Autodesk Inventor part; units mm, degrees
ref_plane "YZ Plane" through (0, 0, 0) normal (1, 0, 0) x (0, 1, 0)
ref_plane "XZ Plane" through (0, 0, 0) normal (0, 1, 0) x (-1, 0, 0)
ref_plane "XY Plane" through (0, 0, 0) normal (0, 0, 1) x (1, 0, 0)
sketch "スケッチ2" plane through (0, 0, 0) normal (0, 0, 1) x (1, 0, 0)
  circle A0 centre (24.8946, 24.5696) radius 0.85
  circle A1 centre (3.8946, 24.5696) radius 0.85
  circle A2 centre (3.8946, 3.5696) radius 0.85
  circle A3 centre (24.8946, 24.5696) radius 2.5
  circle A4 centre (24.8946, 24.5696) radius 1.1
  circle A5 centre (3.8946, 24.5696) radius 1.1
  circle A6 centre (3.8946, 24.5696) radius 2.5
  circle A7 centre (3.8946, 3.5696) radius 2.5
  circle A8 centre (3.8946, 3.5696) radius 1.1
  line L0 (24.8946, 27.0696) -> (3.8946, 27.0696)
  line L1 (24.8946, 22.0696) -> (3.8946, 22.0696)
  line L2 (6.3946, 24.5696) -> (6.3946, 3.5696)
  line L3 (3.8946, 27.0696) -> (-21.1054, 27.0696)
  arc A9 (-21.1054, 27.0696) -> (-56.0009, 1.0696) centre (-21.1054, -9.3477) ccw
  line L4 (3.8946, 1.0696) -> (-56.0009, 1.0696) construction
  circle A10 centre (-53.6054, 0.3545) radius 2.5
  arc A11 (1.5492, 2.7041) -> (-51.1781, -0.2441) centre (-24.3623, -6.8571) ccw
  circle A12 centre (-25.9042, 23.7232) radius 3 construction
  circle A13 centre (-53.6054, 0.3545) radius 1.1
  circle A14 centre (-25.9042, 23.7232) radius 1.1
  circle A15 centre (-43.3948, 16.3537) radius 2.3971 construction
  line L5 (-43.3948, 16.3537) -> (-25.9042, 23.7232) construction
  line L6 (-43.3948, 16.3537) -> (-53.6054, 0.3545) construction
  circle A16 centre (-43.3948, 16.3537) radius 1.1
  point P0 (0, 0)
  point P1 (3.8946, 1.0696)
  point P2 (1.4587, 3.0071)
  point P3 (-51.2099, 1.0696)
  point P4 (-55.9852, 1.6541)
  point P5 (6.3946, 22.0696)
  point P6 (-25.9042, 20.719)
  dimension "d10" = 5
  dimension "d11" = 2.2
  dimension "d12" = 2.2
  dimension "d13" = 5
  dimension "d14" = 5
  dimension "d15" = 2.2
  dimension "d16" = 25
  dimension "d17" = 5
  dimension "d21" = 60
  dimension "d23" = 6
  dimension "d24" = 2.2
  dimension "d25" = 2.2
  dimension "d26" = 2.2
extrude "押し出し1" add sketch "スケッチ2" along normal blind 1.5 contours A3 | A3 L1 L2 A6 L0 | A6 | A6 L1 L2 A7 A11 A10 A9 L3 | L1 A6 L2 | A7 | A10
fillet "フィレット1" radius 2 1 edges at (6.3946, 22.0696, 0.75)
sketch "スケッチ3" plane through (0, 0, 1.5) normal (0, 0, 1) x (1, 0, 0)
  line L0 (-24.3623, 22.7621) -> (4.3946, 22.7621)
  line L1 (4.3946, 22.7621) -> (4.3946, 6.0191)
  line L2 (6.3946, 3.5696) -> (6.3946, 20.0696)
  line L3 (24.8946, 27.0696) -> (-21.1054, 27.0696)
  circle A0 centre (3.8946, 24.5696) radius 1.1
  circle A1 centre (3.8946, 24.5696) radius 2.5
  arc A2 (1.5492, 2.7041) -> (-51.1781, -0.2441) centre (-24.3623, -6.8571) ccw
  arc A3 (1.5492, 2.7041) -> (6.3946, 3.5696) centre (3.8946, 3.5696) ccw
  circle A4 centre (3.8946, 3.5696) radius 2.5
  arc A5 (3.4255, 3.3965) -> (-53.12, 0.2347) centre (-24.3623, -6.8571) ccw
  arc A6 (3.4255, 3.3965) -> (4.3946, 3.5696) centre (3.8946, 3.5696) ccw
  line L4 (4.3946, 3.5696) -> (4.3946, 20.0696)
  point P0 (0, 0)
  point P1 (2.4919, 5.639)
  point P2 (4.3946, 22.1201)
  point P3 (2.1675, 22.7621)
  dimension "d27" = 2
  dimension "d30" = 2
extrude "押し出し2" cut sketch "スケッチ3" against normal through all contours L0 A1 L1 A4 A5
fillet "フィレット2" radius 2 5 edges at (-24.3623, 22.7621, 0.75) (2.4919, 5.639, 0.75) (4.3946, 6.0191, 0.75) (4.3946, 22.1201, 0.75) (2.1675, 22.7621, 0.75)
sketch "スケッチ4" plane through (0, 0, 1.5) normal (0, 0, 1) x (1, 0, 0)
  circle A0 centre (-15.7592, 24.9158) radius 1.1
  circle A1 centre (-0.7592, 24.9158) radius 1.1
  circle A2 centre (-0.7592, 24.9158) radius 2.1538
  line L0 (24.8946, 27.0696) -> (-21.1054, 27.0696)
  line L1 (-8.969, 22.7621) -> (1.4961, 22.7621)
  line L2 (1.3946, 24.5696) -> (1.3946, 3.5696)
  point P0 (0, 0)
  dimension "d34" = 2.2
  dimension "d35" = 2.2
  dimension "d36" = 15
extrude "押し出し3" cut sketch "スケッチ4" against normal through all contours A0 | A1
properties part number "tesaki" material "アルミニウム 2014-T4"
Source: CAD feature listing. Evaluate the final solid. Frame: model axes, mm. A direction names the side the tool comes from. Round coordinates to 2 decimals unless told otherwise and drop trailing zeros. Loops run counter-clockwise (first coordinate to the right, second up) from the corner with the lowest first, then second, coordinate; pieces in that order, holes last. Notation, with made-up numbers: M -0.75,7 L 49.25,7 A20 cw 49.25,25 Z; hole C 51,58 d5. An arc over 180 degrees is marked long. Use a Markdown table: item, result. Add a question column.
1. Line query: line 1 (X direction, y = 23.75, z = 0.5); line 2 (X direction, y = 16, z = 0.6); line 3 (X direction, y = 11, z = 0.5). Output: solid intervals per line, ascending.
2. Section query A-A on y = 13.75. Return the cut outline in (x, z), then the cut area to 3 significant figures.
3. Mould query, pull axis Y, two halves, no side actions, for faces 4 (the flat face through (2, 27.07, 1)), 5 (the cylindrical face through (4.486, 23.642, 0.74)), 6 (the cylindrical face through (-3.909, 14.567, 0.76)), 7 (the cylindrical face through (6.996, 21.499, 0.76)). Classes: pulls with the +Y half, pulls with the -Y half, needs draft (parallel to the pull), parting line crosses it, or undercut.
4. Reachability of faces 1 (the flat face through (-17.6, 20.1, 0)), 2 (the flat face through (17, 22.07, 1)), 3 (the flat face through (-4, 22.762, 1)) from +Z, -Z, +X, -X, +Y, -Y: full face, straight path, thin tool, end or side. Return the list, or none.
5. Section query C-C on z = 1. Give the number of separate pieces and of enclosed holes in the cut face, then the cut area to 3 significant figures.
6. Section query B-B on x = -7.5. Return the cut outline in (y, z), then the cut area to 3 significant figures.
7. Contact query for a flat-ended pin moving along its axis: P1, Ø12, axis at x = -32.5, y = 10.5, coming from the +Z side. Output: stop coordinate, or through.
8. Section query D-D on x = -29.5. Return the cut outline in (y, z), then the cut area to 3 significant figures.
Reported:
| question | item | result |
|---|---|---|
| 1 | line 1 | x = -36.3 to -27, -24.8 to 3.16, 4.63 to 24.16, 25.63 to 27.26 |
| 1 | line 2 | x = -47.25 to -44.44, -42.35 to -39.87, -8.86 to -5.52, 4.39 to 6.39 |
| 1 | line 3 | x = -51.31 to -45.43, -3.29 to -0.73, 4.39 to 6.39 |
| 2 | outline | M -49.26,0 L -42.75,0 L -42.75,1.5 L -49.26,1.5 Z; M -5.97,0 L -3.09,0 L -3.09,1.5 L -5.97,1.5 Z; M 4.39,0 L 6.39,0 L 6.39,1.5 L 4.39,1.5 Z |
| 2 | area | 17.1 mm² |
| 3 | face 4 | pulls with the +Y half |
| 3 | face 5 | undercut |
| 3 | face 6 | undercut |
| 3 | face 7 | pulls with the -Y half |
| 4 | face 1 | -Z, +X, -X, +Y, -Y |
| 4 | face 2 | +Z, -Z, +X, -Y |
| 4 | face 3 | +Z, -Z |
| 5 | separate pieces | 1 |
| 5 | enclosed holes | 9 |
| 5 | area | 562 mm² |
| 6 | outline | M 15.02,0 L 17.49,0 L 17.49,1.5 L 15.02,1.5 Z; M 22.76,0 L 27.07,0 L 27.07,1.5 L 22.76,1.5 Z |
| 6 | area | 10.2 mm² |
| 7 | P1 | passes through |
| 8 | outline | M 20.28,0 L 26.09,0 L 26.09,1.5 L 20.28,1.5 Z |
| 8 | area | 8.71 mm² |
